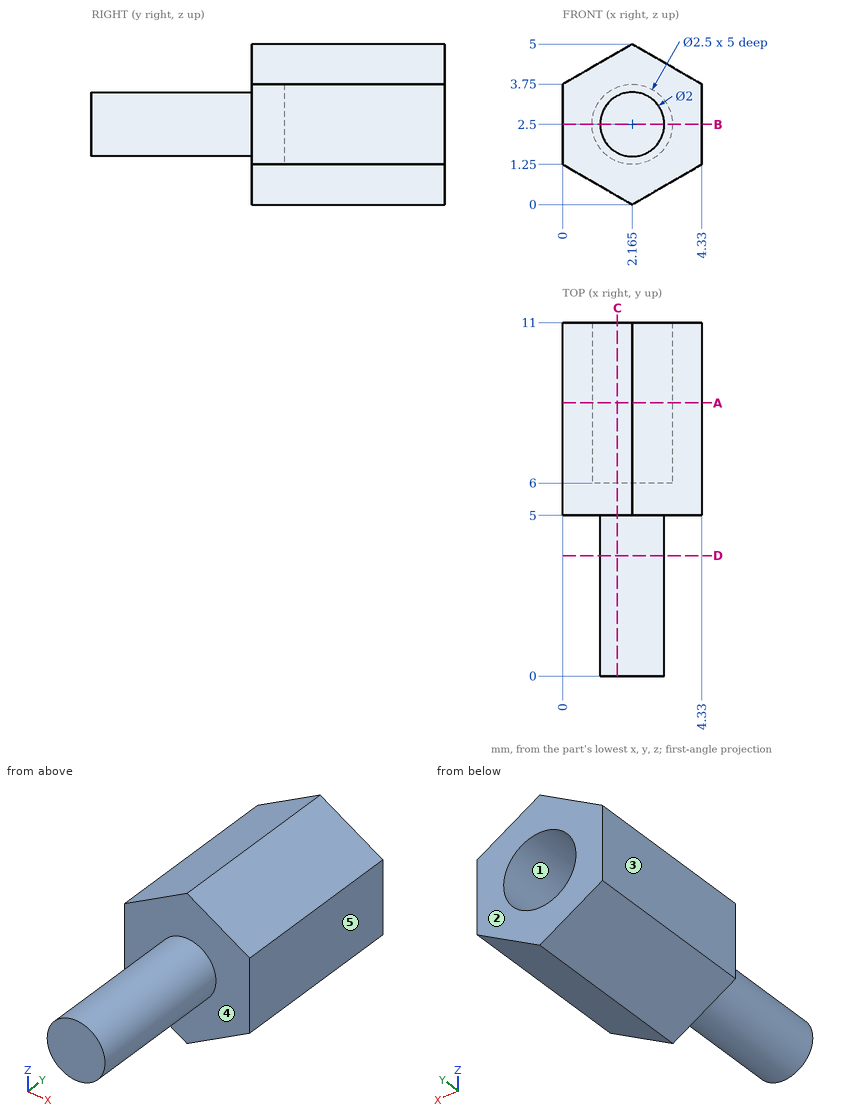
Here's the drawing with two shaded views (mm, measured from the low corner). I have some questions. A direction names the side the tool comes from. Give positions to 0.01 mm unless a question says otherwise; leave off trailing zeros. Write each loop counter-clockwise with the first axis right and the second up, starting at its lowest first coordinate (ties: lowest second). Pieces come first, ordered by that corner, then holes. Notation, with made-up numbers: (82, 79) -> (128, 79) arc R12 ccw to (128, 91) -> close; hole circle Ø10 at (-25, 52). An arc over 180 degrees is marked (long way). Use one line per item in the form item = value. Start each with the question number.
1. Imagine slicing it at B-B on z = 2.5. List the corners of the cut face in (x, y) for me (3 decimals).
2. Imagine slicing it at A-A on y = 8.5. List the corners of the cut face in (x, z) for me (3 decimals), plus the area to 3 significant figures.
3. Imagine slicing it at D-D on y = 3.75. List the corners of the cut face in (x, z) for me (3 decimals).
4. If I drill on L1, parallel to X at y = 8.7, z = 2.5 (3 decimals); L2, parallel to Y at x = 2.8, z = 4.2; L3, parallel to Y at x = 1.9, z = 2, over which ranges is the centre line in solid material (lowest first)?
5. Imagine slicing it at C-C on x = 1.7. List the corners of the cut face in (y, z) for me.
6. Will these pins go through, and if not, where does the flat tip stop? pin 1 Ø0.8 at (x, z) = (2, 2) entering from +Y; pin 2 Ø1 at (y, z) = (8.5, 4.5) entering from +X.
7. Thinking about a two-plate mould opening in X: for the marked faces 1, 2 and 3, which applies, +X half, -X half, draft (parallel to the pull), parting line (faces both ways), or undercut?
8. On a 3-axis mill with a long thin cutter (end or side, diameter ignored), from which of +Z, -Z, +X, -X, +Y, -Y can I reach the whole of each face in a straight line? I mean the marked faces 4 and 5. Say none if no direction works.
Entries:
q1.outline = (0, 5) -> (1.165, 5) -> (1.165, 0) -> (3.165, 0) -> (3.165, 5) -> (4.33, 5) -> (4.33, 11) -> (3.415, 11) -> (3.415, 6) -> (0.915, 6) -> (0.915, 11) -> (0, 11) -> close
q2.outline = (0, 1.25) -> (2.165, 0) -> (4.33, 1.25) -> (4.33, 3.75) -> (2.165, 5) -> (0, 3.75) -> close; hole circle Ø2.5 at (2.165, 2.5)
q2.area = 11.3 mm²
q3.outline = circle Ø2 at (2.165, 2.5)
q4.L1 = 0 to 0.915, 3.415 to 4.33
q4.L2 = 5 to 11
q4.L3 = 0 to 6
q5.outline = (0, 1.61) -> (5, 1.61) -> (5, 0.27) -> (11, 0.27) -> (11, 1.34) -> (6, 1.34) -> (6, 3.66) -> (11, 3.66) -> (11, 4.73) -> (5, 4.73) -> (5, 3.39) -> (0, 3.39) -> close
q6.pin_1 = 6
q6.pin_2 = 3.9
q7.face_1 = undercut
q7.face_2 = draft
q7.face_3 = -X half
q8.face_4 = -Y
q8.face_5 = +Z, -Z, +X, +Y, -Y
